Input: part model. Units: mm. Frame: model coordinates. Face numbers are marked on the shaded views. A direction names the side the tool comes from. Give positions to 0.01 mm unless a question says otherwise; leave off trailing zeros. Order: outer loops, then holes, each group sorted by start corner. A loop starts at its lowest first (then second) coordinate and runs counter-clockwise, first axis right, second up.
```python
from build123d import *

# Parameters (mm, degrees)
EXTRUDE_1_DEPTH        = 50
CUT_EXTRUDE_1_DEPTH    = 45
CUT_EXTRUDE_3_DEPTH    = 274.308913017
PATTERN_LINEAR_3_DEPTH = 5


# Read off the part's stored shape, not the designer's step: 阵列(线性)3
with BuildPart() as part:
    # 草图1 → 凸台-拉伸1 (new body)
    with BuildSketch(Plane(origin=(0, 0, 0), x_dir=(1, 0, 0), z_dir=(0, 1, 0))):
        with BuildLine():
            Line((1.496016616, 189.994110262), (0, 0))
            Line((0, 0), (190, 0))
            ThreePointArc((190, 0), (134.878173099, 133.820321407), (1.496016616, 189.994110262))
        make_face()
    extrude(amount=EXTRUDE_1_DEPTH)

    # 草图2 → 切除-拉伸1 (cut)
    with BuildSketch(Plane(origin=(0, 50, 0), x_dir=(1, 0, 0), z_dir=(0, 1, 0))):
        with BuildLine():
            Line((5.039525077, 5), (184.932420089, 5))
            ThreePointArc((184.932420089, 5), (131.328747491, 130.298734001), (6.455960656, 184.887318581))
            Line((6.455960656, 184.887318581), (5.039525077, 5))
        make_face()
    extrude(amount=-CUT_EXTRUDE_1_DEPTH, mode=Mode.SUBTRACT)

    # 草图3 → 切除-拉伸3 (cut, through all)
    with BuildSketch(Plane.XZ):
        with BuildLine():
            Line((11.494321842, -39.528128563), (39.617406911, -11.182730076))
            ThreePointArc((39.617406911, -11.182730076), (45.274217322, -11.160459514), (45.296487884, -16.817269924))
            Line((45.296487884, -16.817269924), (17.173402815, -45.162668411))
            ThreePointArc((17.173402815, -45.162668411), (11.516592404, -45.184938973), (11.494321842, -39.528128563))
        make_face()
    extrude(amount=-CUT_EXTRUDE_3_DEPTH, mode=Mode.SUBTRACT)

    # 阵列(线性)3 outline → 阵列(线性)3 (cut)
    with BuildSketch(Plane(origin=(0, 0, 0), x_dir=(1, 0, 0), z_dir=(0, 1, 0))):
        with BuildLine():
            ThreePointArc((17.395235092, 73.335367655), (11.738424681, 73.357638217), (11.71615412, 67.700827806))
            Line((11.71615412, 67.700827806), (67.790979496, 11.182730076))
            ThreePointArc((67.790979496, 11.182730076), (73.447789906, 11.160459514), (73.470060469, 16.817269924))
            Line((73.470060469, 16.817269924), (17.395235092, 73.335367655))
        make_face()
        with BuildLine():
            ThreePointArc((18.060731925, 157.853465386), (12.403921514, 157.875735948), (12.381650952, 152.218925537))
            Line((12.381650952, 152.218925537), (152.311697253, 11.182730076))
            ThreePointArc((152.311697253, 11.182730076), (157.968507663, 11.160459514), (157.990778225, 16.817269924))
            Line((157.990778225, 16.817269924), (18.060731925, 157.853465386))
        make_face()
        with BuildLine():
            ThreePointArc((17.61706737, 101.508066899), (11.960256959, 101.530337461), (11.937986397, 95.87352705))
            Line((11.937986397, 95.87352705), (95.964552082, 11.182730076))
            ThreePointArc((95.964552082, 11.182730076), (101.621362492, 11.160459514), (101.643633054, 16.817269924))
            Line((101.643633054, 16.817269924), (17.61706737, 101.508066899))
        make_face()
        with BuildLine():
            ThreePointArc((17.838899648, 129.680766142), (12.182089237, 129.703036704), (12.159818675, 124.046226293))
            Line((12.159818675, 124.046226293), (124.138124667, 11.182730076))
            ThreePointArc((124.138124667, 11.182730076), (129.794935077, 11.160459514), (129.81720564, 16.817269924))
            Line((129.81720564, 16.817269924), (17.838899648, 129.680766142))
        make_face()
    extrude(amount=PATTERN_LINEAR_3_DEPTH, mode=Mode.SUBTRACT)


solid = part.part
```
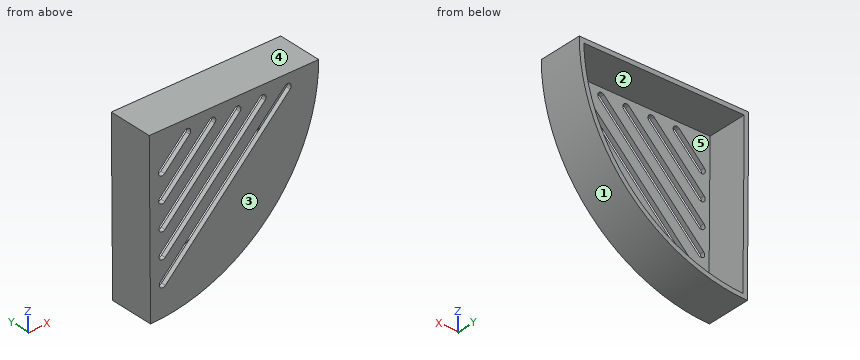
1) Reachability of the marked faces 4 and 5 from +Z, -Z, +X, -X, +Y, -Y: full face, straight path, thin tool, end or side. Return the list, or none.
2) Cut plane C-C (y = 41). Return the cut outline in (x, z).
3) Cut plane A-A (z = -14). Return the cut outline in (x, y), then the cut area to 3 significant figures.
4) First-contact query: P1, Ø1, axis at x = 67.5, y = 25.5, coming from the -Z side; P2, Ø5, axis at x = 75, z = -43, coming from the +Y side; P3, Ø8, axis at y = 19.5, z = -92, coming from the -X side. Flat tips, straight axial feed; report the tip coordinate or a pass-through.
5) Pull-direction query (X, two-part tool) for the marked faces 1, 2 and 3; classes: pulls with the +X half, pulls with the -X half, needs draft (parallel to the pull), parting line crosses it, or undercut.
6) Cut plane B-B (z = -60). Return the cut outline in (x, y), then the cut area to 3 significant figures.
7) Line query: probe 1 along Y at (x, z) = (129, -111); probe 2 along X at (y, z) = (36.5, -157.5); probe 3 along X at (y, z) = (38.5, -134.5). Output: solid intervals per line, ascending.
Geometry says:
1. face 4: +Z, +X, -X, +Y, -Y
1. face 5: +Y
2. outline: (0, 0) - (1.5, -189.99) arc R190 ccw to (190, 0) - close; hole (5.04, -5) - (6.46, -184.89) arc R185 ccw to (184.93, -5) - close
3. outline: (0.11, 0) - (36.82, 0) - (36.82, 5) - (5.11, 5) - (5.11, 50) - (0.11, 50) - close; (46.46, 0) - (65, 0) - (65, 5) - (46.46, 5) - close; (74.63, 0) - (93.17, 0) - (93.17, 5) - (74.63, 5) - close; (102.8, 0) - (121.34, 0) - (121.34, 5) - (102.8, 5) - close; (130.98, 0) - (149.52, 0) - (149.52, 5) - (130.98, 5) - close; (159.15, 0) - (189.48, 0) - (189.48, 50) - (184.47, 50) - (184.47, 5) - (159.15, 5) - close
3. area: 1,160 mm2
4. P1: stops at z = -177.79
4. P2: stops at y = 5
4. P3: stops at x = 0.69
5. face 1: pulls with the +X half
5. face 2: undercut
5. face 3: needs draft
6. outline: (0.47, 0) - (19.36, 0) - (19.36, 5) - (5.47, 5) - (5.47, 50) - (0.47, 50) - close; (30.63, 0) - (47.53, 0) - (47.53, 5) - (30.63, 5) - close; (58.8, 0) - (75.7, 0) - (75.7, 5) - (58.8, 5) - close; (86.97, 0) - (103.88, 0) - (103.88, 5) - (86.97, 5) - close; (115.15, 0) - (180.28, 0) - (180.28, 50) - (175, 50) - (175, 5) - (115.15, 5) - close
6. area: 1,140 mm2
7. probe 1: y = 0 to 5
7. probe 2: x = 1.24 to 6.24, 97.05 to 106.27
7. probe 3: x = 1.06 to 6.06, 127.02 to 134.2
